Part model, mm, in its own coordinate system. A direction names the side the tool comes from. Give positions to 0.01 mm unless a question says otherwise; leave off trailing zeros. Order: outer loops, then holes, each group sorted by start corner. A loop starts at its lowest first (then second) coordinate and runs counter-clockwise, first axis right, second up. Notation, with made-up numbers: (57, 40.25) -> (70, 40.25) arc R25 cw to (70, 58.25) -> close; hole circle Ø8 at (22.5, 37.25). An arc over 180 degrees is marked (long way). Write item = value, one per line. Start each with the question number.
Item 1: Tool access for faces 4 (the face through (0, 0, 405)), 5 (the face through (-8, -8, 400)), 6 (the face through (8, -8, 0)), 7 (the face through (8, 8, 400)): list every direction of +Z, -Z, +X, -X, +Y, -Y with a clear straight run to the whole face (end or side of a thin tool).
Item 2: Flat gauge pins, fed straight in: P1, Ø3, axis at x = -1, y = 0, coming from the +Z side; P2, Ø4, axis at y = 6.5, z = 187.5, coming from the +X side; P3, Ø2, axis at x = 8, z = 195.5, coming from the +Y side; P4, Ø8, axis at y = 0, z = 420, coming from the +X side. Where does each tip first touch, or does it go through?
Item 3: Drill centre lines: line 1 along Z through (x, y) = (2.75, 0.5); line 2 along Y through (x, z) = (7.75, 420); line 3 along Z through (x, y) = (9, 8.5). Where is each one in solid material? Low to high.
Item 4: Pull direction Z, two halves, no side cores. Call faces 1 (the face through (0, 0, -20)), 2 (the face through (-8, -8, 0)), 3 (the face through (-10, 0, 415)): +Z half, -Z half, draft (parallel to the pull), parting line (faces both ways), or undercut.
Item 5: Band-saw the part on B-B on z = 130. Write the cut outline in (x, y), plus the area to 3 significant figures.
Item 6: Band-saw the part on A-A on z = -10. Write the cut outline in (x, y), plus the area to 3 significant figures.
```python
from build123d import *

# Parameters (mm, degrees)
SKIZZE1_R                       = 10
AUFSATZ_LINEAR_AUSTRAGEN1_DEPTH = 400
SKIZZE2_W                       = 20
SKIZZE2_H                       = 20
AUFSATZ_LINEAR_AUSTRAGEN2_DEPTH = 20
SKIZZE3_R                       = 5
SCHNITT_LINEAR_AUSTRAGEN1_DEPTH = 30
SKIZZE4_W                       = 20
SKIZZE4_H                       = 20
AUFSATZ_LINEAR_AUSTRAGEN3_DEPTH = 30
SKIZZE5_W                       = 10
SKIZZE5_H                       = 20
SCHNITT_LINEAR_AUSTRAGEN2_DEPTH = 25
FASE1_SIZE                      = 5
SKIZZE6_R                       = 2.5
SCHNITT_LINEAR_AUSTRAGEN3_DEPTH = 25


with BuildPart() as part:
    # Skizze1 → Aufsatz-Linear austragen1 (new body)
    with BuildSketch(Plane.XY):
        Circle(SKIZZE1_R)
    extrude(amount=AUFSATZ_LINEAR_AUSTRAGEN1_DEPTH)

    # Skizze2 → Aufsatz-Linear austragen2 (add)
    with BuildSketch(Plane(origin=(0, 0, 0), x_dir=(-1, 0, 0), z_dir=(0, 0, -1))):
        Rectangle(SKIZZE2_W, SKIZZE2_H)
    extrude(amount=AUFSATZ_LINEAR_AUSTRAGEN2_DEPTH)

    # Skizze3 → Schnitt-Linear austragen1 (cut)
    with BuildSketch(Plane(origin=(10, 0, 0), x_dir=(0, 0, -1), z_dir=(1, 0, 0))):
        with Locations(Location((10, 0, 0), (0, 0, 90))):
            Circle(SKIZZE3_R)
    extrude(amount=-SCHNITT_LINEAR_AUSTRAGEN1_DEPTH, mode=Mode.SUBTRACT)

    # Skizze4 → Aufsatz-Linear austragen3 (add)
    with BuildSketch(Plane.XY.offset(400)):
        Rectangle(SKIZZE4_W, SKIZZE4_H)
    extrude(amount=AUFSATZ_LINEAR_AUSTRAGEN3_DEPTH)

    # Skizze5 → Schnitt-Linear austragen2 (cut)
    with BuildSketch(Plane.XY.offset(430)):
        Rectangle(SKIZZE5_W, SKIZZE5_H)
    extrude(amount=-SCHNITT_LINEAR_AUSTRAGEN2_DEPTH, mode=Mode.SUBTRACT)

    # Fase1
    fase1_edges = [part.edges().sort_by_distance(p)[0] for p in [
        (0, -10, 405),
        (0, 10, 405),
    ]]
    chamfer(fase1_edges, length=FASE1_SIZE - 0.0001)  # a hair under: the kernel refuses the full size

    # Skizze6 → Schnitt-Linear austragen3 (cut)
    with BuildSketch(Plane(origin=(10, 0, 0), x_dir=(0, 0, -1), z_dir=(1, 0, 0))):
        with Locations((-420, 0)):
            Circle(SKIZZE6_R)
    extrude(amount=-SCHNITT_LINEAR_AUSTRAGEN3_DEPTH, mode=Mode.SUBTRACT)


solid = part.part
```
Values found:
q1.face_4 = +Z, +Y, -Y
q1.face_5 = -X, -Y
q1.face_6 = +X, -Y
q1.face_7 = +X, +Y
q2.P1 = 405
q2.P2 = 8.93
q2.P3 = 7.14
q2.P4 = 10
q3.line_1 = -20 to -14.97, -5.03 to 405
q3.line_2 = -10 to -2.5, 2.5 to 10
q3.line_3 = -20 to 0, 400 to 430
q4.face_1 = -Z half
q4.face_2 = undercut
q4.face_3 = draft
q5.outline = circle Ø20 at (0, 0)
q5.area = 314 mm^2
q6.outline = (-10, -10) -> (10, -10) -> (10, -5) -> (-10, -5) -> close; (-10, 5) -> (10, 5) -> (10, 10) -> (-10, 10) -> close
q6.area = 200 mm^2
